from build123d import *

# Parameters (mm, degrees)
SKETCH1_W           = 21
SKETCH1_H           = 12
BOSS_EXTRUDE1_DEPTH = 60
SKETCH2_R           = 2.25
BOSS_EXTRUDE2_DEPTH = 10
SKETCH3_W           = 55
SKETCH3_H           = 18
BOSS_EXTRUDE3_DEPTH = 3
FILLET1_R           = 2
SKETCH4_R           = 1.25
CUT_EXTRUDE1_DEPTH  = 30


with BuildPart() as part:
    # Sketch1 → Boss-Extrude1 (new body)
    with BuildSketch(Plane.XY):
        Polygon((17.509291985, 21.588576814), (-9.490708015, 21.588576814), (-14.490708015, 21.588576814), (-14.490708015, 18.588576814), (-9.490708015, 18.588576814), (-9.490708015, 6.588576814), (-34.490708015, 6.588576814), (-34.490708015, 18.588576814), (-29.490708015, 18.588576814), (-29.490708015, 21.588576814), (-34.490708015, 21.588576814), (-37.490708015, 21.588576814), (-37.490708015, 3.588576814), (17.509291985, 3.588576814), align=None)
        with Locations((4.009291985, 12.588576814)):
            Rectangle(SKETCH1_W, SKETCH1_H, mode=Mode.SUBTRACT)
    extrude(amount=-BOSS_EXTRUDE1_DEPTH)

    # Sketch2 → Boss-Extrude2 (add)
    # profile 1 of 2: a face of its own
    with BuildSketch(Plane(origin=(-5.490708015, 0, 0), x_dir=(0, 0, -1), z_dir=(1, 0, 0))):
        with BuildLine():
            Line((50, 21.588576814), (40.2, 21.588576814))
            Line((40.2, 21.588576814), (40.2, 33.588576814))
            Line((40.2, 33.588576814), (48, 33.588576814))
            ThreePointArc((48, 33.588576814), (49.414213562, 33.002790376), (50, 31.588576814))
            Line((50, 31.588576814), (50, 21.588576814))
        make_face()
        with Locations(Location((43.5, 27.588576814, 0), (0, 0, 90))):
            Circle(SKETCH2_R, mode=Mode.SUBTRACT)
    # profile 2 of 2: a face of its own
    with BuildSketch(Plane(origin=(-5.490708015, 0, 0), x_dir=(0, 0, -1), z_dir=(1, 0, 0))):
        with BuildLine():
            Line((9.8, 21.588576814), (0, 21.588576814))
            Line((0, 21.588576814), (0, 31.588576814))
            ThreePointArc((0, 31.588576814), (0.585786438, 33.002790376), (2, 33.588576814))
            Line((2, 33.588576814), (9.8, 33.588576814))
            Line((9.8, 33.588576814), (9.8, 21.588576814))
        make_face()
        with Locations(Location((6.5, 27.588576814, 0), (0, 0, 90))):
            Circle(SKETCH2_R, mode=Mode.SUBTRACT)
    extrude(amount=BOSS_EXTRUDE2_DEPTH)

    # Sketch3 → Boss-Extrude3 (add)
    with BuildSketch(Plane(origin=(0, 0, -60), x_dir=(-1, 0, 0), z_dir=(0, 0, -1))):
        with Locations((9.990708015, 12.588576814)):
            Rectangle(SKETCH3_W, SKETCH3_H)
    extrude(amount=BOSS_EXTRUDE3_DEPTH)

    # Fillet1
    fillet1_edges = [part.edges().sort_by_distance(p)[0] for p in [
        (17.509291985, 3.588576814, -31.5),
        (-37.490708015, 3.588576814, -31.5),
        (-37.490708015, 21.588576814, -31.5),
        (17.509291985, 21.588576814, -31.5),
        (4.509291985, 21.588576814, -45.1),
        (-0.490708015, 21.588576814, -50),
        (4.509291985, 21.588576814, -4.9),
        (17.509291985, 12.588576814, -63),
        (-9.990708015, 3.588576814, -63),
        (-37.490708015, 12.588576814, -63),
        (-9.990708015, 21.588576814, -63),
    ]]
    fillet(fillet1_edges, radius=FILLET1_R)

    # Sketch4 → Cut-Extrude1 (cut)
    with BuildSketch(Plane(origin=(17.509291985, 0, 0), x_dir=(0, 0, -1), z_dir=(1, 0, 0))):
        with Locations(Location((22, 12.588576814, 0), (0, 0, 270))):
            Circle(SKETCH4_R)
    extrude(amount=-CUT_EXTRUDE1_DEPTH, mode=Mode.SUBTRACT)


solid = part.part
Work out the finished part from the listing and answer in its coordinate system (mm). A direction names the side the tool comes from. Give positions to 0.01 mm unless a question says otherwise; leave off trailing zeros. Loops run counter-clockwise (first coordinate to the right, second up) from the corner with the lowest first, then second, coordinate; pieces in that order, holes last. Notation, with made-up numbers: (2.5, 31.25) -> (40.5, 31.25) arc R14 cw to (40.5, 54.25) -> close; hole circle Ø6 at (-16.75, -11). An arc over 180 degrees is marked (long way). Use a Markdown table: item, result. Add a question column.
1) Each of these flat-tipped pins is pushed along its axis until it touches: P1, Ø3, axis at y = 28, z = -4, coming from the +X side; P2, Ø4.5, axis at x = -23.5, y = 14.5, coming from the +Z side; P3, Ø9.5, axis at y = 29.5, z = -45, coming from the -X side; P4, Ø10, axis at x = -31, y = 29, coming from the -Z side. Where does it stop, or does it pass through?
2) Which of the six approach directions +Z, -Z, +X, -X, +Y, -Y give full straight-line access (tool end or side, diameter ignored) to faces 4 (the flat face through (-1, 28, -50)), 5 (the flat face through (-5.491, 28, -4)), 6 (the flat face through (-12, 18.589, -30))?
3) For a pull along Z with two mould halves and no side action, classify faces 1 (the cylindrical face through (-0.561, 29.735, -5.824)), 2 (the cylindrical face through (-10.35, 4.16, -62.4)), 3 (the flat face through (-34.491, 13, -30)) as +Z half, -Z half, draft (parallel to the pull), parting line (faces both ways), or undercut.
4) The part is cut by section B-B, the plane y = 30.75. Determine the outline of the cut face in (x, z).
5) The part is cut by section C-C, the plane x = -3. Determine the outline of the cut face in (y, z).
6) Consider line 1 along X through (y, z) = (15.25, -38.5); line 2 along X through (y, z) = (19.75, -7.5); line 3 along Y through (x, z) = (1, -6). Determine where each line is inside the solid, lowest interval first.
7) The part is cut by section A-A, the plane z = -6.5. Count the separate pieces of the cut face and the enclosed holes in it, plus the area to 3 significant figures.
8) The part is cut by section D-D, the plane z = -15. Determine the outline of the cut face in (x, y).
Reported:
| question | item | result |
|---|---|---|
| 1 | P1 | stops at x = 4.51 |
| 1 | P2 | stops at z = -60 |
| 1 | P3 | stops at x = -5.49 |
| 1 | P4 | passes through |
| 2 | face 4 | -Z, +X, -X, +Y |
| 2 | face 5 | +Z, -Z, -X, +Y |
| 2 | face 6 | +Z |
| 3 | face 1 | undercut |
| 3 | face 2 | -Z half |
| 3 | face 3 | draft |
| 4 | outline | (-5.49, -50) -> (4.51, -50) -> (4.51, -40.2) -> (-5.49, -40.2) -> close; (-5.49, -9.8) -> (4.51, -9.8) -> (4.51, 0) -> (-5.49, 0) -> close |
| 5 | outline | (3.59, -61) arc R2 ccw to (5.59, -63) -> (19.59, -63) arc R2 ccw to (21.59, -61) -> (21.59, -52) arc R2 cw to (23.59, -50) -> (31.59, -50) arc R2 ccw to (33.59, -48) -> (33.59, -40.2) -> (21.59, -40.2) -> (21.59, -9.8) -> (33.59, -9.8) -> (33.59, -2) arc R2 ccw to (31.59, 0) -> (18.59, 0) -> (18.59, -60) -> (6.59, -60) -> (6.59, 0) -> (3.59, 0) -> close; hole circle Ø4.5 at (27.59, -43.5); hole circle Ø4.5 at (27.59, -6.5) |
| 6 | line 1 | x = -37.49 to -34.49, -9.49 to -6.49, 14.51 to 17.51 |
| 6 | line 2 | x = -37.48 to -29.49, -14.49 to 17.5 |
| 6 | line 3 | y = 3.59 to 6.59, 18.59 to 25.39, 29.78 to 33.59 |
| 7 | separate pieces | 2 |
| 7 | enclosed holes | 1 |
| 7 | area | 465 mm^2 |
| 8 | outline | (-37.49, 5.59) arc R2 ccw to (-35.49, 3.59) -> (15.51, 3.59) arc R2 ccw to (17.51, 5.59) -> (17.51, 19.59) arc R2 ccw to (15.51, 21.59) -> (-14.49, 21.59) -> (-14.49, 18.59) -> (-9.49, 18.59) -> (-9.49, 6.59) -> (-34.49, 6.59) -> (-34.49, 18.59) -> (-29.49, 18.59) -> (-29.49, 21.59) -> (-35.49, 21.59) arc R2 ccw to (-37.49, 19.59) -> close; hole (-6.49, 6.59) -> (14.51, 6.59) -> (14.51, 18.59) -> (-6.49, 18.59) -> close |
